The model under review builds one solid part; all positions refer to its coordinate system, in mm. Round coordinates to 2 decimals unless told otherwise and drop trailing zeros. Write each loop counter-clockwise with the first axis right and the second up, starting at its lowest first coordinate (ties: lowest second). Pieces come first, ordered by that corner, then holes. Notation, with made-up numbers: (-25, 39.5) -> (-19, 39.5) arc R12 ccw to (-19, 49.5) -> close; hole circle Ø5 at (87.5, 47.25). An arc over 180 degrees is marked (long way). Answer in a Markdown table with one row per item. Add a question column.
```python
from build123d import *

# Parameters (mm, degrees)
F0_W           = 60
F0_H           = 12
F1_DEPTH       = 3
F3_D           = 4.5
F3_DEPTH       = 3.4
F3_CSINK_D     = 9.4
F3_CSINK_ANGLE = 90
F3_TIP         = 1.3519363928
F4_SIZE        = 1


with BuildPart() as f1:
    # F0 (on Top) → F1 (new body)
    with BuildSketch(Plane.XY):
        Rectangle(F0_W, F0_H)
    extrude(amount=F1_DEPTH)

    # F3
    with Locations(Plane.XY.offset(3)):
        with Locations((-23, 0), (23, 0)):
            CounterSinkHole(F3_D / 2, F3_CSINK_D / 2, depth=F3_DEPTH, counter_sink_angle=F3_CSINK_ANGLE)
            with Locations((0, 0, -(F3_DEPTH + F3_TIP / 2))):  # 118° drill point
                Cone(0, F3_D / 2, F3_TIP, mode=Mode.SUBTRACT)

    # F4
    f4_edges = [f1.edges().sort_by_distance(p)[0] for p in [
        (30, 6, 1.5),
        (30, -6, 1.5),
        (-30, -6, 1.5),
        (-30, 6, 1.5),
    ]]
    chamfer(f4_edges, length=F4_SIZE)


solid = f1.part
```
1. Add section A-A on y = 0. Write out the cut boundary in (x, z).
2. For L1, parallel to X at y = 0, z = 0.3; L2, parallel to Y at x = 23, z = 0.45; L3, parallel to X at y = -1.25, z = 1.25, list the stretches that pass through material, from the lowest coordinate up.
3. Add section C-C on z = 2.1. Write out the cut boundary in (x, y).
4. Insertion check: pin 1 Ø2 at (x, y) = (-5.5, -0.5) entering from -Z. The pin has a flat end and moves straight along its axis. Give the tip position at first contact, or say it passes through.
5. Add section B-B on x = -23. Write out the cut boundary in (y, z).
6. Mouldability with a two-part tool opening along X and no side actions: class faces 1 (the flat face through (29.5, 5.5, 1.5)), 2 (the cylindrical face through (-25.146, 0.676, 0.271)), 3 (the flat face through (-29.5, 5.5, 1.5)), 4 (the conical face through (-21.12, -1.44, 0.67)) as pulls with the +X half, pulls with the -X half, needs draft (parallel to the pull), parting line crosses it, or undercut.
Filled in:
| question | item | result |
|---|---|---|
| 1 | outline | (-30, 0) -> (-25.25, 0) -> (-25.25, 0.55) -> (-27.7, 3) -> (-30, 3) -> close; (-20.75, 0) -> (20.75, 0) -> (20.75, 0.55) -> (18.3, 3) -> (-18.3, 3) -> (-20.75, 0.55) -> close; (25.25, 0) -> (30, 0) -> (30, 3) -> (27.7, 3) -> (25.25, 0.55) -> close |
| 2 | L1 | -30 to -25.25, -20.75 to 20.75, 25.25 to 30 |
| 2 | L2 | -6 to -2.25, 2.25 to 6 |
| 2 | L3 | -30 to -25.67, -20.33 to 20.33, 25.67 to 30 |
| 3 | outline | (-30, -5) -> (-29, -6) -> (29, -6) -> (30, -5) -> (30, 5) -> (29, 6) -> (-29, 6) -> (-30, 5) -> close; hole circle Ø7.6 at (-23, 0); hole circle Ø7.6 at (23, 0) |
| 4 | pin 1 | z = 0 |
| 5 | outline | (-6, 0) -> (-2.25, 0) -> (-2.25, 0.55) -> (-4.7, 3) -> (-6, 3) -> close; (2.25, 0) -> (6, 0) -> (6, 3) -> (4.7, 3) -> (2.25, 0.55) -> close |
| 6 | face 1 | pulls with the +X half |
| 6 | face 2 | undercut |
| 6 | face 3 | pulls with the -X half |
| 6 | face 4 | undercut |
